Autodesk Inventor part; units mm, degrees
ref_plane "YZ Plane" through (0, 0, 0) normal (1, 0, 0) x (0, 1, 0)
ref_plane "XZ Plane" through (0, 0, 0) normal (0, 1, 0) x (-1, 0, 0)
ref_plane "XY Plane" through (0, 0, 0) normal (0, 0, 1) x (1, 0, 0)
sketch "Sketch1" plane through (0, 0, 0) normal (0, 0, 1) x (1, 0, 0)
  circle A0 centre (0, 0) radius 42
  circle A1 centre (0, 0) radius 65
  line L0 (45.9619, -45.9619) -> (-45.9619, 45.9619) construction
  line L1 (-45.9619, -45.9619) -> (45.9619, 45.9619) construction
  point P0 (0, 42)
  dimension "d44" = 84
  dimension "d23" = 130
extrude "Plate1" add sketch "Sketch1" along normal blind 3
sketch "Sketch6" plane through (0, 0, 0) normal (0, 0, 1) x (1, 0, 0)
  line L0 (0, 0) -> (0, 55) construction
  circle A0 centre (0, 0) radius 55 construction
  line L1 (0, 0) -> (38.8909, 38.8909) construction
  circle A1 centre (38.8909, 38.8909) radius 5.5
  dimension "d42" = 72.5
  dimension "d32" = 11
  dimension "d33" = 110
  dimension "d34" = 45
extrude "Cut2" cut sketch "Sketch6" along normal blind 3
pattern_circular "Circular Pattern2" count 4 over 360 about axis through (0, 0, -10) along (0, 0, -1) of "Cut2"
equation "\"d35\" = Thickness"
equation "\"d2\" = Thickness"
equation "\"BendRadius\" = Thickness"
equation "\"BendReliefWidth\" = Thickness"
equation "\"BendReliefDepth\" = 0.5 * Thickness"
equation "\"CornerReliefSize\" = 4 * Thickness"
equation "\"MinimumRemnant\" = 2 * Thickness"
equation "\"TransitionRadius\" = BendRadius"
equation "\"JacobiRadiusSize\" = BendRadius"
equation "\"GapSize\" = Thickness"
equation "\"Octaeder_side\" = d41"
equation "\"Octaeder_flange_lenth\" = d42"
properties part number "DSB 138 head loose flange"
Here's how the part is built. I have some questions about the finished solid (model axes, mm). Coordinates: 2 decimals unless noted, no trailing zeros. Order: outer loops, then holes, each group sorted by start corner. A loop starts at its lowest first (then second) coordinate and runs counter-clockwise, first axis right, second up. Notation, with made-up numbers: M 82.25,71.5 L 127.25,71.5 A19 cw 127.25,77.5 Z; hole C -33,0 d6. An arc over 180 degrees is marked long. Answer as a JSON object with one key per item and string values. Group by question number.
(1) I need wall thicknesses on probe 1 along Y at (x, z) = (0, 1.9); probe 2 along X at (y, z) = (28, 1.65). Which ranges of each line are inside material? Lowest first, please.
(2) Suppose I cut it at A-A, the plane x = 0. Please give me the cut outline in (y, z).
(3) If we mould it in two halves opening along X, with no side actions, what happens to faces 1 (the face through (42.4, 0.9, 0)), 2 (the face through (38.17, 33.44, 1.48)), 3 (the face through (62, -19.52, 1.48))? For each: released by +X, released by -X, zero draft, split by the parting line, or undercut.
(4) Suppose I cut it at D-D, the plane y = 56. Please give me the cut outline in (x, z).
(5) Suppose I cut it at C-C, the plane z = 1.1. Please give me the cut outline in (x, y).
Values found:
{
 "1": {"probe 1": "y = -65 to -42, 42 to 65", "probe 2": "x = -58.66 to -31.3, 31.3 to 58.66"},
 "2": {"outline": "M -65,0 L -42,0 L -42,3 L -65,3 Z; M 42,0 L 65,0 L 65,3 L 42,3 Z"},
 "3": {"face 1": "zero draft", "face 2": "undercut", "face 3": "split by the parting line"},
 "4": {"outline": "M -33,0 L 33,0 L 33,3 L -33,3 Z"},
 "5": {"outline": "C 0,0 d130; hole C -38.89,-38.89 d11; hole C -38.89,38.89 d11; hole C 0,0 d84; hole C 38.89,-38.89 d11; hole C 38.89,38.89 d11"}
}
